Input: part model. Units: mm. Frame: model coordinates. Round coordinates to 2 decimals unless told otherwise and drop trailing zeros. Use CSV: the item, a comma, the result in double quotes.
```python
from build123d import *

# Parameters (mm, degrees)
F1_DEPTH = 19.05
F2_R     = 5.08


with BuildPart() as f1:
    # F0 (on Right) → F1 (new body)
    with BuildSketch(Plane.YZ):
        with BuildLine():
            Line((-160.8581324715, 0), (-242.7069797365, 0))
            add(Edge.make_bspline(
                [(-242.7069797365, 0), (-265.2118802071, -74.5986700058), (107.0116907358, 0), (519.2930202635, 0)],
                knots=[0, 0, 0, 0, 762, 762, 762, 762], degree=3))
            Line((519.2930202635, 0), (218.9046558231, 0))
            ThreePointArc((218.9046558231, 0), (207.4913084507, -3.8397523781), (196.0779610783, 0))
            Line((196.0779610783, 0), (150.206251788, 0))
            ThreePointArc((150.206251788, 0), (128.160789609, -10.2089434816), (106.1153274299, 0))
            Line((106.1153274299, 0), (77.678939592, 0))
            ThreePointArc((77.678939592, 0), (53.2129891217, -13.5109411506), (28.7470386513, 0))
            Line((28.7470386513, 0), (-12.8924874617, 0))
            ThreePointArc((-12.8924874617, 0), (-38.6368222535, -15.7596921502), (-64.3811570453, 0))
            Line((-64.3811570453, 0), (-103.0457951603, 0))
            ThreePointArc((-103.0457951603, 0), (-103.0449853734, -0.1249209702), (-103.0447154427, -0.2498442734))
            ThreePointArc((-103.0447154427, -0.2498442734), (-132.0768871191, -29.1568227159), (-160.8581324715, 0))
        make_face()
        with BuildLine():
            add(Edge.make_bspline(
                [(519.2930202635, 0), (269.2858278751, 28.3039230853), (0, 114.9312928319), (-242.7069797365, 0)],
                knots=[0, 0, 0, 0, 762, 762, 762, 762], degree=3))
            Line((-242.7069797365, 0), (-160.8581324715, 0))
            ThreePointArc((-160.8581324715, 0), (-131.9519638159, 28.6574040998), (-103.0457951603, 0))
            Line((-103.0457951603, 0), (-64.3811570453, 0))
            ThreePointArc((-64.3811570453, 0), (-45.3981508389, 41.2529550685), (-9.7295738803, 13.147556223))
            ThreePointArc((-9.7295738803, 13.147556223), (-10.5314234079, 6.3862276376), (-12.8924874617, 0))
            Line((-12.8924874617, 0), (28.7470386513, 0))
            ThreePointArc((28.7470386513, 0), (45.2009450137, 43.1710467842), (82.1202374948, 15.3963072225))
            ThreePointArc((82.1202374948, 15.3963072225), (80.9877286834, 7.3842631146), (77.678939592, 0))
            Line((77.678939592, 0), (106.1153274299, 0))
            ThreePointArc((106.1153274299, 0), (118.2019905399, 45.8359416643), (157.0680379821, 18.6983048916))
            ThreePointArc((157.0680379821, 18.6983048916), (155.2984263817, 8.7395058225), (150.206251788, 0))
            Line((150.206251788, 0), (196.0779610783, 0))
            ThreePointArc((196.0779610783, 0), (199.0938059623, 31.9551771791), (226.3738016805, 15.0427408516))
            ThreePointArc((226.3738016805, 15.0427408516), (224.4037447781, 6.6452383633), (218.9046558231, 0))
            Line((218.9046558231, 0), (519.2930202635, 0))
        make_face()
    extrude(amount=F1_DEPTH)

    # F2
    f2_edges = [f1.edges().sort_by_distance(p)[0] for p in [
        (9.525, -242.70698, 0),
    ]]
    fillet(f2_edges, radius=F2_R)


solid = f1.part
```
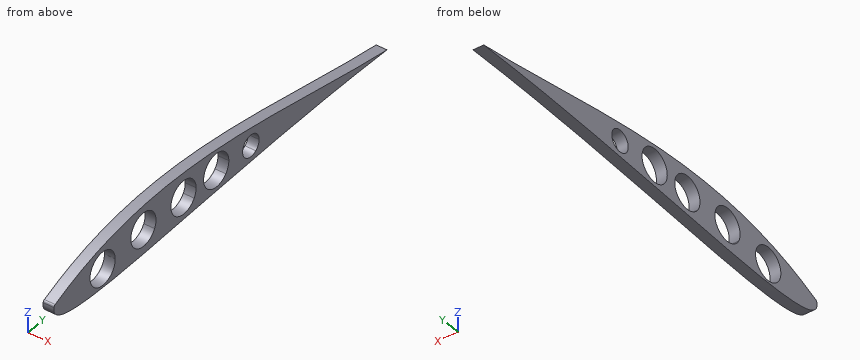
Item 1: Line query: line 1 (Z direction, x = 12, y = 62); line 2 (Z direction, x = 8.5, y = -20.5); line 3 (Z direction, x = 13.75, y = -95). Output: solid intervals per line, ascending.
Worked answers:
line 1,"z = -21.82 to -12.14, 42.94 to 57.73"
line 2,"z = -27.69 to -9.36, 35.66 to 55.88"
line 3,"z = -31.91 to 46.72"
Item 2: First-contact query: pin 1 Ø4 at (x, y) = (10.5, 411) entering from +Z; pin 2 Ø5 at (x, y) = (5, -128.5) entering from -Z. Flat tips, straight axial feed; report the tip coordinate or a pass-through.
Worked answers:
pin 1,"stops at z = 15.27"
pin 2,"stops at z = -33.02"
Item 3: Section query A-A on x = 9.25. Give the number of separate pieces and of enclosed holes in the cut face, plus the area to 3 significant figures.
Worked answers:
separate pieces,"1"
enclosed holes,"5"
area,"28,200 mm²"
